```python
from build123d import *

# Parameters (mm, degrees)
F0_W      = 120
F0_H      = 73
F1_DEPTH  = 1
F2_W      = 2
F2_H      = 73
F3_DEPTH  = 261
F4_W      = 120
F4_H      = 73
F5_DEPTH  = 2
F6_W      = 1.8
F6_H      = 73
F7_DEPTH  = 260
F9_W      = 1.8
F9_H      = 73
F10_DEPTH = 190
F11_W     = 60
F11_H     = 73
F11_W_2   = 1.8
F12_DEPTH = 1.8


with BuildPart() as f1:
    # F0 (on Top) → F1 (new body)
    with BuildSketch(Plane.XY):
        with Locations((-40, 36.5)):
            Rectangle(F0_W, F0_H)
    extrude(amount=F1_DEPTH)

    # F2 (on face) → F3 (join)
    with BuildSketch(Plane.XY.offset(1)):
        with Locations((-99, 36.5)):
            Rectangle(F2_W, F2_H)
        with Locations((19, 36.5)):
            Rectangle(F2_W, F2_H)
    extrude(amount=F3_DEPTH)

    # F4 (on face) → F5 (join)
    with BuildSketch(Plane.XY.offset(262)):
        with Locations((-40, 36.5)):
            Rectangle(F4_W, F4_H)
    extrude(amount=F5_DEPTH)

    # F6 (on face) → F7 (join)
    with BuildSketch(Plane.XY.offset(1)):
        with Locations((-97.1, 36.5)):
            Rectangle(F6_W, F6_H)
        with Locations((17.1, 36.5)):
            Rectangle(F6_W, F6_H)
    extrude(amount=F7_DEPTH)

    # F9 (on face) → F10 (join)
    with BuildSketch(Plane.XY.offset(1)):
        with Locations((-35.3, 36.5)):
            Rectangle(F9_W, F9_H)
    extrude(amount=F10_DEPTH)

    # F11 (on face) → F12 (join)
    with BuildSketch(Plane.XY.offset(191)):
        with Locations((-66.2, 36.5)):
            Rectangle(F11_W, F11_H)
        with Locations((-35.3, 36.5)):
            Rectangle(F11_W_2, F11_H)
    extrude(amount=F12_DEPTH)


solid = f1.part
```
Could you check a few things on this model? Use its own coordinates, in mm. A direction names the side the tool comes from. Give positions to 0.01 mm unless a question says otherwise; leave off trailing zeros. Order: outer loops, then holes, each group sorted by start corner. A loop starts at its lowest first (then second) coordinate and runs counter-clockwise, first axis right, second up.
Q1. For faces 4 (the flat face through (-35, 73, 122)), 5 (the flat face through (-66, 37, 192.8)), which set-ups out of +Z, -Z, +X, -X, +Y, -Y let a thin tool reach every point of the face, with its end or its side?
Q2. Suppose I cut it at C-C, the plane y = 54.5. Write out the boundary of the cut face in (x, z), and give its area (3 significant figures).
Q3. I'm going to push a flat-ended pin straight in: P1, Ø3, axis at x = -66.5, y = 41, coming from the -Z side. Where does the tip first touch, or does it pass through?
Q4. Suppose I cut it at B-B, the plane z = 181. Write out the boundary of the cut face in (x, y).
Q5. Suppose I cut it at A-A, the plane x = -73.5. Write out the boundary of the cut face in (y, z).
Q6. We'd pull the mould along Z, two halves only. Please class faces 1 (the flat face through (-41, 37, 264)), 2 (the flat face through (20, 36, 130)), 3 (the flat face through (-96.2, 36, 226)): +Z half, -Z half, draft (parallel to the pull), parting line (faces both ways), or undercut.
Q7. Suppose I cut it at D-D, the plane x = -16.5. Write out the boundary of the cut face in (y, z).
Q8. If I drill on line 1 along Z through (x, y) = (-91.5, 61); line 2 along X through (y, z) = (9.5, 164); line 3 along X through (y, z) = (64, 242.5), over which ranges is the centre line in solid material (lowest first)?
Solution:
1. face 4: +Z, -Z, +X, -X, +Y
1. face 5: +Y, -Y
2. outline: (-100, 0) - (20, 0) - (20, 264) - (-100, 264) - close; hole (-98, 261) - (-96.2, 261) - (-96.2, 192.8) - (-34.4, 192.8) - (-34.4, 1) - (16.2, 1) - (16.2, 261) - (18, 261) - (18, 262) - (-98, 262) - close; hole (-96.2, 1) - (-36.2, 1) - (-36.2, 191) - (-96.2, 191) - close
2. area: 2,790 mm2
3. P1: stops at z = 0
4. outline: (-100, 0) - (-96.2, 0) - (-96.2, 73) - (-100, 73) - close; (-36.2, 0) - (-34.4, 0) - (-34.4, 73) - (-36.2, 73) - close; (16.2, 0) - (20, 0) - (20, 73) - (16.2, 73) - close
5. outline: (0, 0) - (73, 0) - (73, 1) - (0, 1) - close; (0, 191) - (73, 191) - (73, 192.8) - (0, 192.8) - close; (0, 262) - (73, 262) - (73, 264) - (0, 264) - close
6. face 1: +Z half
6. face 2: draft
6. face 3: undercut
7. outline: (0, 0) - (73, 0) - (73, 1) - (0, 1) - close; (0, 262) - (73, 262) - (73, 264) - (0, 264) - close
8. line 1: z = 0 to 1, 191 to 192.8, 262 to 264
8. line 2: x = -100 to -96.2, -36.2 to -34.4, 16.2 to 20
8. line 3: x = -100 to -96.2, 16.2 to 20
